```python
from build123d import *

# Parameters (mm, degrees)
BASENUTSKE_R  = 3.96875
BASENUT_DEPTH = 8.5598


with BuildPart() as part:
    # BaseNutSke → BaseNut (new body)
    with BuildSketch(Plane.XY):
        Polygon((8.7376, 5.044655712), (8.7376, -5.044655712), (0, -10.089311424), (-8.7376, -5.044655712), (-8.7376, 5.044655712), (0, 10.089311424), align=None)
        Circle(BASENUTSKE_R, mode=Mode.SUBTRACT)
    extrude(amount=-BASENUT_DEPTH)

    # Sketch3 → Double-Chamfer (revolve, cut)
    with BuildSketch(Plane(origin=(0, 0, 0), x_dir=(0, 0, -1), z_dir=(1, 0, 0))):
        Polygon((8.5598, 7.1374), (7.44855, 10.089311424), (7.44855, 22.789311424), (21.2598, 22.789311424), (21.2598, 7.1374), align=None)
        Polygon((1.11125, 22.789311424), (-12.7, 22.789311424), (-12.7, 7.1374), (0, 7.1374), (1.11125, 10.089311424), align=None)
    revolve(axis=Axis((0, 0, 0), (0, 0, -1)), mode=Mode.SUBTRACT)

    # Sketch5 → EndChamfer (revolve, cut)
    with BuildSketch(Plane(origin=(0, 0, 0), x_dir=(0, 0, -1), z_dir=(1, 0, 0))):
        Polygon((8.5344, 5.55625), (7.311662586, 3.81), (8.5852, 3.81), (8.5852, 5.55625), align=None)
        Polygon((-0.0508, 5.55625), (0, 5.55625), (1.222737414, 3.81), (-0.0508, 3.81), align=None)
    revolve(axis=Axis((0, 0, -25.037505729), (0, 0, -1)), mode=Mode.SUBTRACT)


solid = part.part
```
Could you check a few things on this model? Use its own coordinates, in mm. Round coordinates to 2 decimals unless told otherwise and drop trailing zeros. Loops run counter-clockwise (first coordinate to the right, second up) from the corner with the lowest first, then second, coordinate; pieces in that order, holes last.
Q1. Please list where these lines run through material, in increasing order: L1, parallel to X at y = 0, z = -3; L2, parallel to X at y = -3.5, z = -1.5; L3, parallel to Y at x = -1.5, z = -3.5.
Q2. Thinking about a two-plate mould opening in X: for faces 1 (the flat face through (0, -6, 0)), 2 (the flat face through (-4.43, 7.53, -4.23)), 3 (the cylindrical face through (3.785, 1.192, -4.223)), 4 (the flat face through (4.31, 7.6, -4.23)), which applies, pulls with the +X half, pulls with the -X half, needs draft (parallel to the pull), parting line crosses it, or undercut?
Q3. For P1, Ø2, axis at x = -4, z = -2, coming from the -Y side; P2, Ø1, axis at x = 6, y = -5.5, coming from the -Z side; P3, Ø2, axis at x = -4, z = -4, coming from the +Y side, each with a flat end and sliding along its axis, tell me the tip position at first contact or that it passes through.
Q4. I want a section at B-B (z = -1.5). Write out the boundary of the cut face in (x, y), and give its area (3 significant figures).
Answer below:
1. L1: x = -8.74 to -3.97, 3.97 to 8.74
1. L2: x = -8.74 to -1.87, 1.87 to 8.74
1. L3: y = -9.22 to -3.67, 3.67 to 9.22
2. face 1: needs draft
2. face 2: pulls with the -X half
2. face 3: undercut
2. face 4: pulls with the +X half
3. P1: stops at y = -8.36
3. P2: stops at z = -8.37
3. P3: stops at y = 8.36
4. outline: (-8.74, -5.04) - (0, -10.09) - (8.74, -5.04) - (8.74, 5.04) - (0, 10.09) - (-8.74, 5.04) - close; hole circle Ø7.94 at (0, 0)
4. area: 215 mm2
